Can you work these out from the drawing? Everything is in mm from the part's minimum corner. Give positions to 0.01 mm unless a question says otherwise; leave off trailing zeros. Loops run counter-clockwise (first coordinate to the right, second up) from the corner with the lowest first, then second, coordinate; pieces in that order, holes last. Notation, with made-up numbers: M 49,47 L 80,47 A26 ccw 80,61 Z; hole C 15.5,73.5 d4. An arc over 180 degrees is marked long. Use CSV: the item, a comma, the result in double quotes.
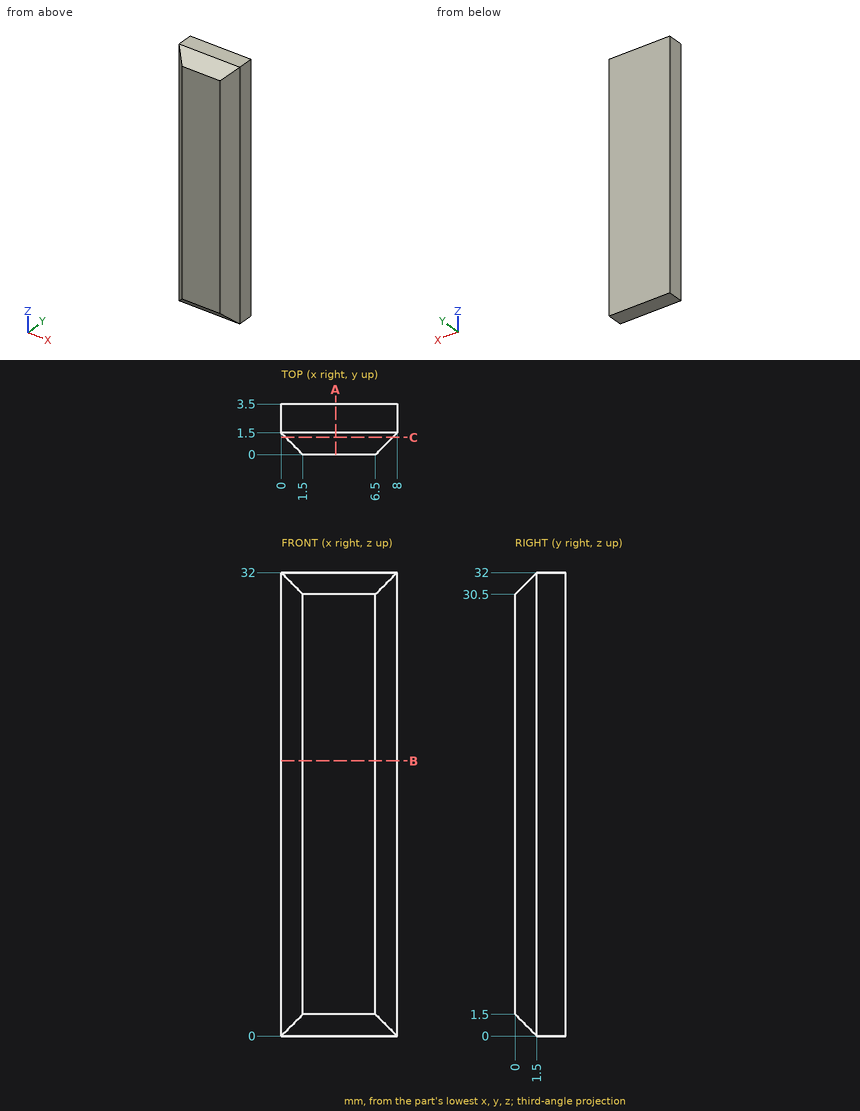
Q1. I want a section at B-B, the plane z = 19. Please give me the cut outline in (x, y), then the cut area to 4 significant figures.
Model answer:
outline,"M 0,1.5 L 1.5,0 L 6.5,0 L 8,1.5 L 8,3.5 L 0,3.5 Z"
area,"25.75 mm2"
Q2. I want a section at C-C, the plane y = 1.2. Please give me the cut outline in (x, z).
Model answer:
outline,"M 0.3,0.3 L 7.7,0.3 L 7.7,31.7 L 0.3,31.7 Z"
Q3. Please list where these lines run through material, in increasing order: L1, parallel to Z at x = 6, y = 0.7; L2, parallel to Y at x = 5.75, z = 1; L3, parallel to X at y = 0.65, z = 8.5. Write a range as from..to.
Model answer:
L1,"0.8..31.2"
L2,"0.5..3.5"
L3,"0.85..7.15"
Q4. I want a section at A-A, the plane x = 3.75. Please give me the cut outline in (y, z).
Model answer:
outline,"M 0,1.5 L 1.5,0 L 3.5,0 L 3.5,32 L 1.5,32 L 0,30.5 Z"
